Can you work these out from the model? Positions are in its coordinate system, mm. A direction names the side the tool comes from. Give positions to 0.01 mm unless a question says otherwise; leave off trailing zeros. Loops run counter-clockwise (first coordinate to the right, second up) from the corner with the lowest first, then second, coordinate; pieces in that order, holes last. Notation, with made-up numbers: (27.25, -30) - (55.25, -30) arc R34 ccw to (55.25, 6) - close; hole circle Ø5 at (37, 24.25). An arc over 180 degrees is marked (long way). Answer in a Markdown table with one row per item.
from build123d import *

# Parameters (mm, degrees)
BOSS_EXTRUDE1_DEPTH = 8
BOSS_EXTRUDE3_DEPTH = 8
CRVPATTERN1_DEPTH   = 8


# Read off the part's stored shape, not the designer's step: CrvPattern1
with BuildPart() as part:
    # Sketch1 → Boss-Extrude1 (new body)
    with BuildSketch(Plane(origin=(0, 0, 0), x_dir=(1, 0, 0), z_dir=(0, 1, 0))):
        with BuildLine():
            Line((-7.606089126, -31.378516667), (-12.870329337, -2.3326))
            ThreePointArc((-12.870329337, -2.3326), (0, 13.08), (12.870329337, -2.3326))
            Line((12.870329337, -2.3326), (7.606089126, -31.378516667))
            ThreePointArc((7.606089126, -31.378516667), (0, -37.73), (-7.606089126, -31.378516667))
        make_face()
        with BuildLine():
            ThreePointArc((-5.638148861, -31.02185), (0, -35.73), (5.638148861, -31.02185))
            Line((5.638148861, -31.02185), (10.902389071, -1.975933333))
            ThreePointArc((10.902389071, -1.975933333), (0, 11.08), (-10.902389071, -1.975933333))
            Line((-10.902389071, -1.975933333), (-5.638148861, -31.02185))
        make_face(mode=Mode.SUBTRACT)
    extrude(amount=BOSS_EXTRUDE1_DEPTH)

    # Sketch2 → Boss-Extrude3 (add)
    with BuildSketch(Plane(origin=(0, 0, 0), x_dir=(1, 0, 0), z_dir=(0, 1, 0))):
        with BuildLine():
            ThreePointArc((-1.165, 11.018583167), (-0.981152237, 10.94243093), (-0.905, 10.758583167))
            ThreePointArc((-0.905, 10.758583167), (0, 9.943845961), (0.905, 10.758583167))
            ThreePointArc((0.905, 10.758583167), (0.981152237, 10.94243093), (1.165, 11.018583167))
            ThreePointArc((1.165, 11.018583167), (0, 11.08), (-1.165, 11.018583167))
        make_face()
    extrude(amount=BOSS_EXTRUDE3_DEPTH)

    # CrvPattern1 outline → CrvPattern1 (add)
    with BuildSketch(Plane(origin=(0, 0, 0), x_dir=(1, 0, 0), z_dir=(0, 1, 0))):
        with BuildLine():
            ThreePointArc((-1.824495283, 10.928751849), (-2.963479144, 10.676337919), (-4.069609665, 10.30556535))
            ThreePointArc((-4.069609665, 10.30556535), (-3.872091938, 10.281359754), (-3.749541755, 10.124577689))
            ThreePointArc((-3.749541755, 10.124577689), (-2.659601093, 9.581575785), (-2.005482944, 10.608683939))
            ThreePointArc((-2.005482944, 10.608683939), (-1.981277348, 10.806201665), (-1.824495283, 10.928751849))
        make_face()
        with BuildLine():
            ThreePointArc((-10.791666914, 0.325671569), (-10.979340539, 0.391836316), (-11.06526029, 0.57132715))
            ThreePointArc((-11.06526029, 0.57132715), (-11.063997012, -0.595289939), (-10.940077478, -1.755307601))
            ThreePointArc((-10.940077478, -1.755307601), (-10.873912731, -1.567633976), (-10.694421897, -1.481714224))
            ThreePointArc((-10.694421897, -1.481714224), (-9.929483935, -0.534248326), (-10.791666914, 0.325671569))
        make_face()
        with BuildLine():
            ThreePointArc((-10.311404493, 3.200167829), (-10.474544311, 3.314117655), (-10.509326889, 3.510049622))
            ThreePointArc((-10.509326889, 3.510049622), (-10.820135393, 2.385596376), (-11.010991108, 1.23469624))
            ThreePointArc((-11.010991108, 1.23469624), (-10.897041283, 1.397836059), (-10.701109316, 1.432618636))
            ThreePointArc((-10.701109316, 1.432618636), (-9.710628125, 2.14097499), (-10.311404493, 3.200167829))
        make_face()
        with BuildLine():
            ThreePointArc((-9.079820232, 5.841489648), (-9.206539356, 5.994921805), (-9.18765039, 6.193018676))
            ThreePointArc((-9.18765039, 6.193018676), (-9.787884177, 5.192660526), (-10.279608785, 4.134736173))
            ThreePointArc((-10.279608785, 4.134736173), (-10.126176628, 4.261455297), (-9.928079758, 4.242566331))
            ThreePointArc((-9.928079758, 4.242566331), (-8.784224959, 4.660200036), (-9.079820232, 5.841489648))
        make_face()
        with BuildLine():
            ThreePointArc((-7.18665129, 8.057181889), (-7.267716561, 8.23891682), (-7.196532361, 8.424744624))
            ThreePointArc((-7.196532361, 8.424744624), (-8.042456481, 7.621370857), (-8.799221359, 6.733506032))
            ThreePointArc((-8.799221359, 6.733506032), (-8.617486428, 6.814571302), (-8.431658623, 6.743387102))
            ThreePointArc((-8.431658623, 6.743387102), (-7.217775126, 6.839868035), (-7.18665129, 8.057181889))
        make_face()
        with BuildLine():
            ThreePointArc((-4.76984, 9.685802142), (-4.799344742, 9.88259806), (-4.681052017, 10.042616791))
            ThreePointArc((-4.681052017, 10.042616791), (-5.71102974, 9.494763784), (-6.677694581, 8.841651151))
            ThreePointArc((-6.677694581, 8.841651151), (-6.480898663, 8.871155893), (-6.320879932, 8.752863168))
            ThreePointArc((-6.320879932, 8.752863168), (-5.125415163, 8.521161417), (-4.76984, 9.685802142))
        make_face()
        with BuildLine():
            ThreePointArc((-5.358787187, -32.02886665), (-4.902775765, -32.965752822), (-4.284641775, -33.804568945))
            ThreePointArc((-4.284641775, -33.804568945), (-4.253283685, -33.672171144), (-4.159348022, -33.573740464))
            ThreePointArc((-4.159348022, -33.573740464), (-3.930645139, -32.377698364), (-5.096173957, -32.025045153))
            ThreePointArc((-5.096173957, -32.025045153), (-5.226962568, -32.062553109), (-5.358787187, -32.02886665))
        make_face()
        with BuildLine():
            ThreePointArc((4.301302835, -33.401557112), (4.399165403, -33.496084492), (4.435884173, -33.627096856))
            ThreePointArc((4.435884173, -33.627096856), (5.019378866, -32.763826296), (5.436895219, -31.809162894))
            ThreePointArc((5.436895219, -31.809162894), (5.306550294, -31.848184784), (5.174343952, -31.816029058))
            ThreePointArc((5.174343952, -31.816029058), (4.024127982, -32.215810168), (4.301302835, -33.401557112))
        make_face()
        with BuildLine():
            ThreePointArc((2.024455519, -35.096408218), (2.061948343, -35.227201168), (2.028246633, -35.359021888))
            ThreePointArc((2.028246633, -35.359021888), (2.965185558, -34.903118865), (3.804073193, -34.28508193))
            ThreePointArc((3.804073193, -34.28508193), (3.671679021, -34.253708522), (3.57325921, -34.159761471))
            ThreePointArc((3.57325921, -34.159761471), (2.377243578, -33.930920208), (2.024455519, -35.096408218))
        make_face()
        with BuildLine():
            ThreePointArc((-0.794764946, -35.425877399), (-0.827686591, -35.557895098), (-0.922779735, -35.655208003))
            ThreePointArc((-0.922779735, -35.655208003), (0.116587527, -35.728813782), (1.15209953, -35.612981977))
            ThreePointArc((1.15209953, -35.612981977), (1.053125917, -35.519618539), (1.01486035, -35.389049577))
            ThreePointArc((1.01486035, -35.389049577), (0.093470356, -34.592894948), (-0.794764946, -35.425877399))
        make_face()
        with BuildLine():
            ThreePointArc((-3.401059435, -34.301696362), (-3.495575491, -34.399569865), (-3.626583606, -34.436303793))
            ThreePointArc((-3.626583606, -34.436303793), (-2.763245543, -35.019698603), (-1.808533841, -35.4371045))
            ThreePointArc((-1.808533841, -35.4371045), (-1.847570812, -35.30676409), (-1.815430382, -35.174554029))
            ThreePointArc((-1.815430382, -35.174554029), (-2.215344568, -34.02438432), (-3.401059435, -34.301696362))
        make_face()
        with BuildLine():
            ThreePointArc((10.974594379, -1.524689547), (11.074074387, -0.36232095), (11.05078642, 0.804064363))
            ThreePointArc((11.05078642, 0.804064363), (10.968663006, 0.622805134), (10.782423353, 0.552705528))
            ThreePointArc((10.782423353, 0.552705528), (9.938527966, -0.325168205), (10.723235544, -1.25632648))
            ThreePointArc((10.723235544, -1.25632648), (10.904494773, -1.338449894), (10.974594379, -1.524689547))
        make_face()
        with BuildLine():
            ThreePointArc((3.535643905, 10.201243009), (3.654867535, 10.36056937), (3.851832122, 10.388926282))
            ThreePointArc((3.851832122, 10.388926282), (2.738143815, 10.73633869), (1.59410025, 10.964727283))
            ThreePointArc((1.59410025, 10.964727283), (1.753426611, 10.845503653), (1.781783523, 10.648539065))
            ThreePointArc((1.781783523, 10.648539065), (2.457371869, 9.635424017), (3.535643905, 10.201243009))
        make_face()
        with BuildLine():
            ThreePointArc((6.135279783, 8.883944999), (6.292773656, 9.005579053), (6.490146906, 8.980222333))
            ThreePointArc((6.490146906, 8.980222333), (5.509951663, 9.612847272), (4.468672705, 10.138903504))
            ThreePointArc((4.468672705, 10.138903504), (4.590306759, 9.981409631), (4.564950039, 9.784036381))
            ThreePointArc((4.564950039, 9.784036381), (4.944955829, 8.627136509), (6.135279783, 8.883944999))
        make_face()
        with BuildLine():
            ThreePointArc((8.287879594, 6.919334403), (8.472168203, 6.994413506), (8.655568872, 6.917190724))
            ThreePointArc((8.655568872, 6.917190724), (7.880286848, 7.788933123), (7.017643405, 8.574326857))
            ThreePointArc((7.017643405, 8.574326857), (7.092722508, 8.390038247), (7.015499725, 8.206637579))
            ThreePointArc((7.015499725, 8.206637579), (7.072234526, 6.990248301), (8.287879594, 6.919334403))
        make_face()
        with BuildLine():
            ThreePointArc((9.836598048, 4.450559019), (10.034253538, 4.473612668), (10.190318466, 4.350150522))
            ThreePointArc((10.190318466, 4.350150522), (9.676439183, 5.397492448), (9.055286209, 6.38499739))
            ThreePointArc((9.055286209, 6.38499739), (9.078339857, 6.187341901), (8.954877712, 6.031276973))
            ThreePointArc((8.954877712, 6.031276973), (8.684207644, 4.844028293), (9.836598048, 4.450559019))
        make_face()
        with BuildLine():
            ThreePointArc((10.668590575, 1.657501702), (10.865211135, 1.626850133), (10.982568934, 1.46614447))
            ThreePointArc((10.982568934, 1.46614447), (10.767535277, 2.612773248), (10.43313196, 3.730436636))
            ThreePointArc((10.43313196, 3.730436636), (10.402480392, 3.533816076), (10.241774729, 3.416458277))
            ThreePointArc((10.241774729, 3.416458277), (9.663421677, 2.344856923), (10.668590575, 1.657501702))
        make_face()
    extrude(amount=CRVPATTERN1_DEPTH)


solid = part.part
Q1. On a 3-axis mill with a long thin cutter (end or side, diameter ignored), from which of +Z, -Z, +X, -X, +Y, -Y can I reach the whole of each face in a straight line? I mean faces 3 (the face through (-5.523, 3.944, 31.525)), 4 (the face through (-10.2, 3.94, 17.06)). Say none if no direction works.
Checked values:
| item | result |
|---|---|
| face 3 | +Y, -Y |
| face 4 | +Z, -X, +Y, -Y |
Q2. If we mould it in two halves opening along Z, with no side actions, what happens to faces 1 (the face through (9.94, 3.94, 0.31)), 2 (the face through (10.275, 3.944, 16.652))? For each: released by +Z, released by -Z, zero draft, split by the parting line, or undercut.
Checked values:
| item | result |
|---|---|
| face 1 | undercut |
| face 2 | released by +Z |
Q3. If I drill on line 1 (X direction, y = 7, z = 30.5); line 2 (X direction, y = 5.5, z = 20.5); line 3 (X direction, y = 2, z = 36.5), over which ranges is the centre line in solid material (lowest first)? Write a range as [from, to].
Checked values:
| item | result |
|---|---|
| line 1 | x = [-7.77, -5.73], [5.73, 7.77] |
| line 2 | x = [-9.58, -7.55], [7.55, 9.58] |
| line 3 | x = [-4.18, 4.18] |
Q4. Imagine slicing it at A-A, the plane z = 0.5. Write out the boundary of the cut face in (x, y).
Checked values:
| item | result |
|---|---|
| outline | (-13.07, 0) - (-9.93, 0) - (-9.93, 8) - (-13.07, 8) - close; (9.95, 0) - (13.07, 0) - (13.07, 8) - (9.95, 8) - close |
Q5. Imagine slicing it at B-B, the plane x = -2.5. Write out the boundary of the cut face in (y, z), and give its area (3 significant figures).
Checked values:
| item | result |
|---|---|
| outline | (0, -12.84) - (8, -12.84) - (8, -9.64) - (0, -9.64) - close; (0, 33.92) - (8, 33.92) - (8, 37.31) - (0, 37.31) - close |
| area | 52.7 mm² |
Q6. For pin 1 (4 mm diameter, centred on y = 5, z = 2.5, fed in from -X); pin 2 (4 mm diameter, centred on x = 5.5, y = 3, fed in from +Z); pin 3 (4 mm diameter, centred on x = -2.5, y = 3, fed in from -Z), each with a flat end and sliding along its axis, tell me the tip position at first contact or that it passes through.
Checked values:
| item | result |
|---|---|
| pin 1 | stops at x = -13.07 |
| pin 2 | stops at z = 36.89 |
| pin 3 | stops at z = -13.07 |
